from build123d import *

# Parameters (mm, degrees)
F1_DEPTH = 76.2
F2_R     = 16.022792
F3_DEPTH = 76.2


with BuildPart() as f1:
    # F0 (on Front) → F1 (new body)
    with BuildSketch(Plane.XZ):
        Polygon((-43.420587, -22.448728), (-44.851206, -39.973821), (55.292182, -39.973821), (55.292182, -22.448728), (5.935797, -22.448728), (5.935797, 17.787455), (55.292182, 17.787455), (55.292182, 33.34545), (-35.015699, 33.34545), (-43.420587, 33.34545), (-43.420587, 21.900488), (-6.224472, 21.900488), (-6.224472, -22.448728), align=None)
    extrude(amount=F1_DEPTH)

    # F2 (on face) → F3 (cut)
    with BuildSketch(Plane.YZ.offset(5.935797)):
        with Locations((-45.915954, -3.561358)):
            Circle(F2_R)
    extrude(amount=-F3_DEPTH, mode=Mode.SUBTRACT)


solid = f1.part
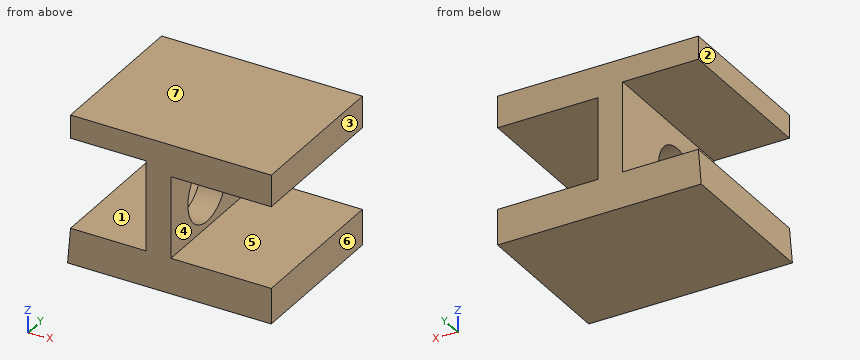
The model under review builds one solid part; all positions refer to its coordinate system, in mm. Face numbers are marked on the shaded views. A direction names the side the tool comes from. Give positions to 0.01 mm unless a question says otherwise; leave off trailing zeros. Order: outer loops, then holes, each group sorted by start corner. A loop starts at its lowest first (then second) coordinate and runs counter-clockwise, first axis right, second up. Notation, with made-up numbers: M 65,84 L 124,84 A18 ccw 124,98 Z; hole C -19,19 d1. An arc over 180 degrees is marked long. One line per question, with ' | ' between items. Start each with the question number.
1) Consider section B-B, the plane y = -65. Give the boundary of the cut face in (x, z), then the cut area to 3 significant figures.
2) Consider section C-C, the plane z = -12. Give the boundary of the cut face in (x, y), then the cut area to 3 significant figures.
3) Consider section D-D, the plane y = -47. Give the boundary of the cut face in (x, z).
4) Consider section A-A, the plane x = 35.5. Give the boundary of the cut face in (y, z).
5) Wall thickness on L1, parallel to Z at x = 13, y = -20.5; L2, parallel to Z at x = -24, y = -68; L3, parallel to X at y = -62, z = -7.5: over which ranges is each line inside the solid? List them lowest first. Write a range as from..to.
6) Mouldability with a two-part tool opening along Z and no side actions: class the marked faces 5, 6 and 7 as pulls with the +Z half, pulls with the -Z half, needs draft (parallel to the pull), parting line crosses it, or undercut.
7) For the marked faces 1, 2, 3 and 4, list the 3-axis set-ups (+Z, -Z, +X, -X, +Y, -Y) from which the entire face can be reached by the end or side of a thin tool; tool diameter is ignored.
8) Clearance check with flat-ended pins moving along their axes: P1, Ø12, axis at y = -35, z = 21.5, coming from the -X side; P2, Ø22, axis at y = -20.5, z = -9, coming from the -X side; P3, Ø12, axis at y = -34.5, z = 1, coming from the +X side. State where each tip first meets the part, or that it passes through.
Found:
1) outline: M -44.85,-39.97 L 55.29,-39.97 L 55.29,-22.45 L 5.94,-22.45 L 5.94,17.79 L 55.29,17.79 L 55.29,33.35 L -43.42,33.35 L -43.42,21.9 L -6.22,21.9 L -6.22,-22.45 L -43.42,-22.45 Z | area: 3,610 mm²
2) outline: M -6.22,-76.2 L 5.94,-76.2 L 5.94,-59.54 L -6.22,-59.54 Z; M -6.22,-32.3 L 5.94,-32.3 L 5.94,0 L -6.22,0 Z | area: 595 mm²
3) outline: M -44.85,-39.97 L 55.29,-39.97 L 55.29,-22.45 L 5.94,-22.45 L 5.94,-19.55 L -6.22,-19.55 L -6.22,-22.45 L -43.42,-22.45 Z; M -43.42,21.9 L -6.22,21.9 L -6.22,12.42 L 5.94,12.42 L 5.94,17.79 L 55.29,17.79 L 55.29,33.35 L -43.42,33.35 Z
4) outline: M -76.2,-39.97 L 0,-39.97 L 0,-22.45 L -76.2,-22.45 Z; M -76.2,17.79 L 0,17.79 L 0,33.35 L -76.2,33.35 Z
5) L1: z = -39.97..-22.45, 17.79..33.35 | L2: z = -39.97..-22.45, 21.9..33.35 | L3: x = -6.22..5.94
6) face 5: undercut | face 6: needs draft | face 7: pulls with the +Z half
7) face 1: -X, +Y, -Y | face 2: +Z, -X, +Y, -Y | face 3: +Z, -Z, +X, +Y, -Y | face 4: +X, +Y, -Y
8) P1: stops at x = -43.42 | P2: stops at x = -6.22 | P3: stops at x = 5.94
